from build123d import *

# Parameters (mm, degrees)
SKETCH_W         = 100
SKETCH_H         = 200
PAD_DEPTH        = 7
HOLE_D           = 5.5
HOLE_CSINK_D     = 11
HOLE_CSINK_ANGLE = 90
SKETCH002_R      = 2.25
HOLE001_DEPTH    = 7.001
SKETCH003_W      = 10
SKETCH003_H      = 5
PAD001_DEPTH     = 10
SKETCH005_W      = 4
SKETCH005_H      = 50
PAD002_DEPTH     = 20
PAD009_DEPTH     = 3
PAD010_DEPTH     = 3
SKETCH019_W      = 13.993252
SKETCH019_H      = 12
PAD011_DEPTH     = 10
SKETCH020_R      = 2
POCKET001_DEPTH  = 14
SKETCH022_W      = 18
SKETCH022_H      = 31
PAD012_DEPTH     = 5
PAD013_DEPTH     = 4
SKETCH024_R      = 2.5
POCKET003_DEPTH  = 7
SKETCH026_W      = 23
SKETCH026_H      = 20
PAD014_DEPTH     = 20
SKETCH034_R      = 2.1
POCKET008_DEPTH  = 120
SKETCH035_W      = 50
SKETCH035_H      = 50
SKETCH035_R      = 11
SKETCH035_R_2    = 1.720547
SKETCH035_R_3    = 1.714858
SKETCH035_R_4    = 2.211749
SKETCH035_R_5    = 1.868355
PAD015_DEPTH     = 7
POCKET_DEPTH     = 7


with BuildPart() as part:
    # Sketch → Pad (new body)
    with BuildSketch(Plane.XY):
        with Locations((0, 100)):
            Rectangle(SKETCH_W, SKETCH_H)
    extrude(amount=PAD_DEPTH)

    # Hole (through all)
    with Locations(Plane.XY.offset(7)):
        with Locations((17, 7), (17, 43), (-17, 43), (-17, 7), (12, 115), (12, 75), (-12, 115), (-12, 75)):
            CounterSinkHole(HOLE_D / 2, HOLE_CSINK_D / 2, counter_sink_angle=HOLE_CSINK_ANGLE)

    # Sketch002 (on Face5 of Hole) → Hole001 (cut, through all)
    with BuildSketch(Plane.XY.offset(7)):
        with Locations((0, 10)):
            Circle(SKETCH002_R)
        with Locations((0, 50)):
            Circle(SKETCH002_R)
        with Locations((0, 90)):
            Circle(SKETCH002_R)
        with Locations((0, 130)):
            Circle(SKETCH002_R)
        with Locations((0, 170)):
            Circle(SKETCH002_R)
    extrude(amount=-HOLE001_DEPTH, mode=Mode.SUBTRACT)

    # Sketch003 (on Face5 of Hole001) → Pad001 (join)
    with BuildSketch(Plane.XY.offset(7)):
        with Locations((-2e-06, 2.5)):
            Rectangle(SKETCH003_W, SKETCH003_H)
    extrude(amount=PAD001_DEPTH)

    # Sketch005 (on DatumPlane) → Pad002 (join)
    with BuildSketch(Plane.XY.offset(7)):
        with Locations((-48, 82)):
            Rectangle(SKETCH005_W, SKETCH005_H)
        with Locations((48, 82)):
            Rectangle(SKETCH005_W, SKETCH005_H)
    extrude(amount=PAD002_DEPTH)

    # Sketch017 (on DatumPlane) → Pad009 (join)
    with BuildSketch(Plane(origin=(0, 107, 0), x_dir=(-1, 0, 0), z_dir=(0, 1, 0))):
        Polygon((46, 7), (46, 27), (36, 7), align=None)
        Polygon((-46, 27), (-46, 7), (-36, 7), align=None)
    extrude(amount=-PAD009_DEPTH)

    # Sketch018 (on DatumPlane) → Pad010 (join)
    with BuildSketch(Plane(origin=(0, 107, 0), x_dir=(-1, 0, 0), z_dir=(0, 1, 0))):
        Polygon((-46, 7), (-46, 27), (-36, 7), align=None)
        Polygon((46, 7), (46, 26.679939), (36, 7), align=None)
    extrude(amount=-PAD010_DEPTH)

    # Sketch019 (on Face5 of Pad010) → Pad011 (join)
    with BuildSketch(Plane.XY.offset(7)):
        with Locations((-28.003374, 31.717157)):
            Rectangle(SKETCH019_W, SKETCH019_H)
    extrude(amount=PAD011_DEPTH)

    # Sketch020 (on DatumPlane) → Pocket001 (cut)
    with BuildSketch(Plane.XZ.offset(-25.717157)):
        with Locations((28, 12)):
            Circle(SKETCH020_R)
    extrude(amount=-POCKET001_DEPTH, mode=Mode.SUBTRACT)

    # Sketch022 → Pad012 (join)
    with BuildSketch(Plane(origin=(0, 200, 0), x_dir=(-1, 0, 0), z_dir=(0, 1, 0))):
        with Locations((0, 15.5)):
            Rectangle(SKETCH022_W, SKETCH022_H)
    extrude(amount=-PAD012_DEPTH)

    # Sketch023 (on DatumPlane) → Pad013 (join)
    with BuildSketch(Plane.YZ.offset(9)):
        Polygon((200, 7), (189, 7), (195, 31), (200, 31), align=None)
    extrude(amount=PAD013_DEPTH)

    # Sketch024 (on Face5 of Pad013) → Pocket003 (cut)
    with BuildSketch(Plane.XY.offset(7)):
        with Locations((0, 189.428879)):
            Circle(SKETCH024_R)
    extrude(amount=-POCKET003_DEPTH, mode=Mode.SUBTRACT)

    # Sketch026 (on DatumPlane) → Pad014 (join)
    with BuildSketch(Plane.YZ.offset(50)):
        with Locations((188.5, 10)):
            Rectangle(SKETCH026_W, SKETCH026_H)
    extrude(amount=PAD014_DEPTH)

    # Sketch034 (on DatumPlane) → Pocket008 (cut)
    with BuildSketch(Plane(origin=(-50, 0, 0), x_dir=(0, -1, 0), z_dir=(-1, 0, 0))):
        with Locations((-99, 17)):
            Circle(SKETCH034_R)
        with Locations((-82, 17)):
            Circle(SKETCH034_R)
        with Locations((-65, 17)):
            Circle(SKETCH034_R)
    extrude(amount=-POCKET008_DEPTH, mode=Mode.SUBTRACT)

    # Sketch035 (on DatumPlane) → Pad015 (join)
    with BuildSketch(Plane.XY.offset(7)):
        with Locations((-25, 225)):
            Rectangle(SKETCH035_W, SKETCH035_H)
        with Locations((-28, 229)):
            Circle(SKETCH035_R, mode=Mode.SUBTRACT)
        with Locations((-43.5, 244.5)):
            Circle(SKETCH035_R_2, mode=Mode.SUBTRACT)
        with Locations((-12.5, 244.5)):
            Circle(SKETCH035_R_3, mode=Mode.SUBTRACT)
        with Locations((-12.5, 213.5)):
            Circle(SKETCH035_R_4, mode=Mode.SUBTRACT)
        with Locations((-43.5, 213.5)):
            Circle(SKETCH035_R_5, mode=Mode.SUBTRACT)
    extrude(amount=-PAD015_DEPTH)

    # Sketch036 (on DatumPlane) → Pocket (cut)
    with BuildSketch(Plane.XY.offset(7)):
        with BuildLine():
            ThreePointArc((-25.4, 20.702306), (-28, 23.302306), (-30.6, 20.702306))
            Line((-30.6, 20.702306), (-30.6, 5.702306))
            ThreePointArc((-30.6, 5.702306), (-28, 3.102306), (-25.4, 5.702306))
            Line((-25.4, 5.702306), (-25.4, 20.702306))
        make_face()
    extrude(amount=-POCKET_DEPTH, mode=Mode.SUBTRACT)


solid = part.part
Work out the finished part from the listing and answer in its coordinate system (mm). A direction names the side the tool comes from. Coordinates: 2 decimals unless noted, no trailing zeros. Write each loop counter-clockwise with the first axis right and the second up, starting at its lowest first coordinate (ties: lowest second). Pieces come first, ordered by that corner, then holes. Notation, with made-up numbers: M -31.75,-26.75 L -1.75,-26.75 A34 cw -1.75,8.25 Z; hole C 0.25,-21.5 d10. An arc over 180 degrees is marked long. Write item = value, one per line.
1. The part is cut by section A-A (y = 90). Determine the outline of the cut face in (x, z), then the cut area to 4 significant figures.
Solution:
outline = M -50,0 L -2.25,0 L -2.25,7 L -46,7 L -46,27 L -50,27 Z; M 2.25,0 L 50,0 L 50,27 L 46,27 L 46,7 L 2.25,7 Z
area = 828.5 mm2
2. The part is cut by section C-C (z = 12.5). State how many separate pieces and enclosed holes the cut face has, then the cut area to 3 significant figures.
Solution:
separate_pieces = 6
enclosed_holes = 0
area = 1,250 mm2
3. For faces 5 (the face through (-9.71, 113.25, 4.38)), 6 (the face through (-27.9, 23.3, 3.5)), 7 (the face through (50, 87, 10)), 8 (the face through (46, 80, 19)), 9 (the face through (41, 106, 17)), determine the directions among +Z, -Z, +X, -X, +Y, -Y from which every point of the face is accessible in a straight line to the end or side of a thin tool.
Solution:
face_5 = +Z
face_6 = +Z, -Z
face_7 = +Z, -Z, +X, -Y
face_8 = +Z, -Y
face_9 = +Z, +Y, -Y
4. The part is cut by section D-D (x = 40). Determine the outline of the cut face in (y, z), then the cut area to 3 significant figures.
Solution:
outline = M 0,0 L 200,0 L 200,7 L 107,7 L 107,15 L 104,15 L 104,7 L 0,7 Z
area = 1,420 mm2
5. Straight lines are drawn through the part: line 1 (Y direction, x = 12, z = 2.95); line 2 (X direction, y = 43, z = 1.7); line 3 (Y direction, x = 17, z = 1). For each, find the intervals that lie inside material, in ascending order. Write a range as from..to.
Solution:
line_1 = 0..72.25, 77.75..112.25, 117.75..200
line_2 = -50..-19.75, -14.25..14.25, 19.75..50
line_3 = 0..4.25, 9.75..40.25, 45.75..200
6. Determine the mould class of faces 1 (the face through (0, 225, 4)), 2 (the face through (-35, 32, 12)), 3 (the face through (0, 195, 19)), 4 (the face through (-19.66, 5.9, 4.38)) for opening direction X: released by +X, released by -X, zero draft, split by the parting line, or undercut.
Solution:
face_1 = released by +X
face_2 = released by -X
face_3 = zero draft
face_4 = undercut
7. Flat-ended cylindrical pins translate along their axes: pin 1 (2.5 mm diameter, centred on y = 2.5, z = 10.5, fed in from +X); pin 2 (1.2 mm diameter, centred on x = 48.5, y = 93.5, fed in from +Z); pin 3 (12 mm diameter, centred on x = 25.5, y = 112.5, fed in from +Z); pin 4 (5 mm diameter, centred on x = 12, y = 75, fed in from +Z). Find the tip coordinate at first contact, or state that the pin passes through.
Solution:
pin_1 = 5
pin_2 = 27
pin_3 = 7
pin_4 = through
8. The part is cut by section B-B (z = 22.5). Determine the outline of the cut face in (x, y) (3 decimals).
Solution:
outline = M -50,57 L -46,57 L -46,104 L -43.75,104 L -43.75,107 L -50,107 Z; M -9,195 L 9,195 L 9,192.875 L 13,192.875 L 13,200 L -9,200 Z; M 43.75,104 L 46,104 L 46,57 L 50,57 L 50,107 L 43.75,107 Z
